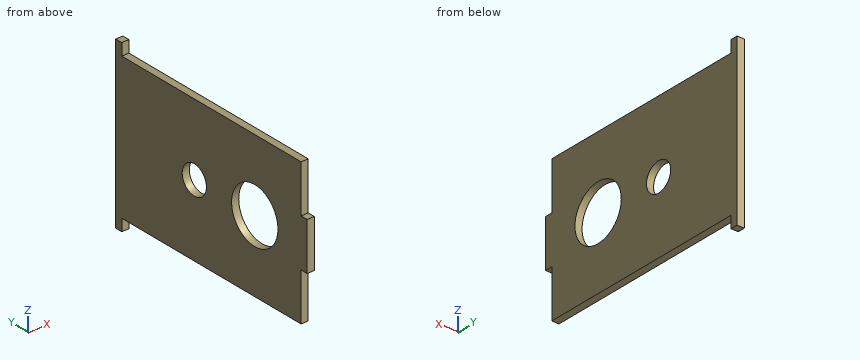
from build123d import *

# Parameters (mm, degrees)
SKETCH1_W           = 60
SKETCH1_H           = 96
BOSS_EXTRUDE1_DEPTH = 3
SKETCH2_R           = 11.5
SKETCH2_R_2         = 6
CUT_EXTRUDE1_DEPTH  = 3
SKETCH3_W           = 5
SKETCH3_H           = 3
SKETCH3_W_2         = 20
BOSS_EXTRUDE2_DEPTH = 3
SKETCH6_W           = 60
SKETCH6_H           = 4
CUT_EXTRUDE2_DEPTH  = 10


with BuildPart() as part:
    # Sketch1 → Boss-Extrude1 (new body)
    with BuildSketch(Plane(origin=(0, 0, 0), x_dir=(0, 0, -1), z_dir=(1, 0, 0))):
        Rectangle(SKETCH1_W, SKETCH1_H)
    extrude(amount=BOSS_EXTRUDE1_DEPTH)

    # Sketch2 → Cut-Extrude1 (cut)
    with BuildSketch(Plane(origin=(3, 0, 0), x_dir=(0, 0, -1), z_dir=(1, 0, 0))):
        with Locations((0, -25)):
            Circle(SKETCH2_R)
        with Locations((0, 5)):
            Circle(SKETCH2_R_2)
    extrude(amount=-CUT_EXTRUDE1_DEPTH, mode=Mode.SUBTRACT)

    # Sketch3 → Boss-Extrude2 (add)
    with BuildSketch(Plane(origin=(0, 0, 0), x_dir=(0, 0, -1), z_dir=(1, 0, 0))):
        with Locations((-32.5, 42.5)):
            Rectangle(SKETCH3_W, SKETCH3_H)
        with Locations((32.5, 42.5)):
            Rectangle(SKETCH3_W, SKETCH3_H)
        with Locations((0, -49.5)):
            Rectangle(SKETCH3_W_2, SKETCH3_H)
    extrude(amount=BOSS_EXTRUDE2_DEPTH)

    # Sketch6 → Cut-Extrude2 (cut)
    with BuildSketch(Plane(origin=(3, 0, 0), x_dir=(0, 0, -1), z_dir=(1, 0, 0))):
        with Locations((0, 46)):
            Rectangle(SKETCH6_W, SKETCH6_H)
    extrude(amount=-CUT_EXTRUDE2_DEPTH, mode=Mode.SUBTRACT)


solid = part.part
Can you work these out from the model? Positions are in its coordinate system, mm. Give positions to 0.01 mm unless a question says otherwise; leave off trailing zeros. Write each loop counter-clockwise with the first axis right and the second up, starting at its lowest first coordinate (ties: lowest second). Pieces come first, ordered by that corner, then holes. Notation, with made-up numbers: (-9, 8.25) -> (8, 8.25) arc R26 cw to (8, 43.25) -> close; hole circle Ø2 at (51.25, 21). An arc over 180 degrees is marked (long way). Answer as a JSON object with one key per item and string values. Group by question number.
Item 1: Suppose I cut it at D-D (y = 5). Please give me the cut outline in (x, z), plus the area to 3 significant figures.
Item 2: Suppose I cut it at C-C (x = 0.95). Please give me the cut outline in (y, z).
Item 3: Suppose I cut it at B-B (z = 0). Please give me the cut outline in (x, y), plus the area to 3 significant figures.
Item 4: I'm going to push flat-ended pins straight in: P1, Ø0.9, axis at x = 1, y = -49.5, coming from the +Z side; P2, Ø3, axis at y = -41, z = 27.5, coming from the -X side; P3, Ø0.9, axis at x = 2, y = -49.5, coming from the -Z side; P4, Ø1.5, axis at x = 1, z = -33, coming from the -Y side. Where does each tip first touch, or does it pass through?
Item 5: Please list where these lines run through material, in increasing order: line 1 (Y direction, x = 2.15, z = 0); line 2 (Z direction, x = 0.2, y = -2); line 3 (Z direction, x = 1.25, y = -25.5). Write a range as [from, to].
Item 6: Suppose I cut it at A-A (y = -25). Please give me the cut outline in (x, z).
Findings:
{
 "1": {"outline": "(0, -30) -> (3, -30) -> (3, -6) -> (0, -6) -> close; (0, 6) -> (3, 6) -> (3, 30) -> (0, 30) -> close", "area": "144 mm²"},
 "2": {"outline": "(-51, -10) -> (-48, -10) -> (-48, -30) -> (41, -30) -> (41, -35) -> (44, -35) -> (44, 35) -> (41, 35) -> (41, 30) -> (-48, 30) -> (-48, 10) -> (-51, 10) -> close; hole circle Ø23 at (-25, 0); hole circle Ø12 at (5, 0)"},
 "3": {"outline": "(0, -51) -> (3, -51) -> (3, -36.5) -> (0, -36.5) -> close; (0, -13.5) -> (3, -13.5) -> (3, -1) -> (0, -1) -> close; (0, 11) -> (3, 11) -> (3, 44) -> (0, 44) -> close", "area": "180 mm²"},
 "4": {"P1": "stops at z = 10", "P2": "stops at x = 0", "P3": "stops at z = -10", "P4": "stops at y = 41"},
 "5": {"line 1": "y = [-51, -36.5], [-13.5, -1], [11, 44]", "line 2": "z = [-30, 30]", "line 3": "z = [-30, -11.49], [11.49, 30]"},
 "6": {"outline": "(0, -30) -> (3, -30) -> (3, -11.5) -> (0, -11.5) -> close; (0, 11.5) -> (3, 11.5) -> (3, 30) -> (0, 30) -> close"}
}
